Build history of the part. All positions in model axes, mm. A direction names the side the tool comes from. Coordinates: 2 decimals unless noted, no trailing zeros. Order: outer loops, then holes, each group sorted by start corner. A loop starts at its lowest first (then second) coordinate and runs counter-clockwise, first axis right, second up. Notation, with made-up numbers: (20.25, 69.25) - (26.25, 69.25) arc R25 cw to (26.25, 107.25) - close; hole circle Ø7 at (71.5, -5). An arc over 180 degrees is marked (long way). One line per item, written item: value.
from build123d import *

# Parameters (mm, degrees)
SKETCH_1_W              = 26
SKETCH_1_H              = 32.5
HOLE_WIZARD_M39_1_D     = 45
HOLE_WIZARD_M39_1_DEPTH = 10
SKETCH_4_R              = 8
EXTRUDE_1_DEPTH         = 10
CUT_EXTRUDE_1_DEPTH     = 5
SKETCH_6_R              = 1.5
CUT_EXTRUDE_2_DEPTH     = 53.80624963
FILLET_1_R              = 5
FILLET_2_R              = 3


with BuildPart() as part:
    # 草图1 → 旋转1 (revolve)
    with BuildSketch(Plane(origin=(0, 0, 0), x_dir=(-1, 0, 0), z_dir=(0, 0, -1)), mode=Mode.PRIVATE) as revolve_1_sk:
        with Locations((-13, 16.25)):
            Rectangle(SKETCH_1_W, SKETCH_1_H)
    revolve(revolve_1_sk.sketch.rotate(Axis((26, 0, 0), (-1, 0, 0)), 270), axis=Axis((26, 0, 0), (-1, 0, 0)))

    # M39 间隙孔1
    with Locations(Plane(origin=(26, 0, 0), x_dir=(0, 0, -1), z_dir=(1, 0, 0))):
        with Locations((0, 0)):
            Hole(HOLE_WIZARD_M39_1_D / 2, depth=HOLE_WIZARD_M39_1_DEPTH)

    # 草图4 → 凸台-拉伸1 (add)
    with BuildSketch(Plane(origin=(16, 0, 0), x_dir=(0, 0, -1), z_dir=(1, 0, 0))):
        with Locations(Location((0, 0, 0), (0, 0, 180))):
            Circle(SKETCH_4_R)
    extrude(amount=EXTRUDE_1_DEPTH)

    # 草图5 → 切除-拉伸1 (cut)
    with BuildSketch(Plane(origin=(26, 0, 0), x_dir=(0, 0, -1), z_dir=(1, 0, 0))):
        Polygon((3.464101615, -6), (6.92820323, 0), (3.464101615, 6), (-3.464101615, 6), (-6.92820323, 0), (-3.464101615, -6), align=None)
    extrude(amount=-CUT_EXTRUDE_1_DEPTH, mode=Mode.SUBTRACT)

    # 草图6 → 切除-拉伸2 (cut, through all)
    with BuildSketch(Plane(origin=(0, 0, 0), x_dir=(0, 0, -1), z_dir=(1, 0, 0))):
        Circle(SKETCH_6_R)
    extrude(amount=CUT_EXTRUDE_2_DEPTH, mode=Mode.SUBTRACT)

    # 圆角1
    fillet_1_edges = [part.edges().sort_by_distance(p)[0] for p in [
        (0, 0, -32.5),
    ]]
    fillet(fillet_1_edges, radius=FILLET_1_R)

    # 圆角2
    fillet_2_edges = [part.edges().sort_by_distance(p)[0] for p in [
        (26, 0, -32.5),
    ]]
    fillet(fillet_2_edges, radius=FILLET_2_R)


solid = part.part
1. Band-saw the part on C-C, the plane x = 3.25. Give the cut face in (y, z), and give its area (3 significant figures).
Values found:
outline: circle Ø64.37 at (0, 0); hole circle Ø3 at (0, 0)
area: 3,250 mm2
2. Two-plate mould, pull along Y, no slides. Class faces 1 (the face through (13.87, 9.76, 31)), 2 (the face through (23.54, -2.96, 5.22)), 3 (the face through (26, -22, 7)): pulls with the +Y half, pulls with the -Y half, needs draft (parallel to the pull), parting line crosses it, or undercut.
Values found:
face 1: parting line crosses it
face 2: undercut
face 3: needs draft
3. Band-saw the part on A-A, the plane z = 0. Give the cut face in (x, y).
Values found:
outline: (0, -27.5) arc R5 ccw to (5, -32.5) - (23, -32.5) arc R3 ccw to (26, -29.5) - (26, -22.5) - (16, -22.5) - (16, -8) - (26, -8) - (26, -6) - (21, -6) - (21, -1.5) - (0, -1.5) - close; (0, 1.5) - (21, 1.5) - (21, 6) - (26, 6) - (26, 8) - (16, 8) - (16, 22.5) - (26, 22.5) - (26, 29.5) arc R3 ccw to (23, 32.5) - (5, 32.5) arc R5 ccw to (0, 27.5) - close
4. 3-axis set-ups, long thin cutter, end or side, ignore diameter. For faces 4 (the face through (24, 6, 0)), 5 (the face through (0, -6, 0)): which of +Z, -Z, +X, -X, +Y, -Y reach the whole face in a straight line?
Values found:
face 4: +X
face 5: +Z, -Z, -X, +Y, -Y
5. Band-saw the part on B-B, the plane x = 11. Give the cut face in (y, z), and give its area (3 significant figures).
Values found:
outline: circle Ø65 at (0, 0); hole circle Ø3 at (0, 0)
area: 3,310 mm2
6. Flat gauge pins, fed straight in: P1, Ø2, axis at x = 20.5, z = 22, coming from the +Y side; P2, Ø10, axis at x = 21.5, z = 10, coming from the +Y side; P3, Ø13.5, axis at y = -10, z = 2, coming from the +X side; P4, Ø1.5, axis at x = 23.5, z = 1, coming from the -Y side. Where does each tip first touch, or does it go through?
Values found:
P1: stops at y = 24.8
P2: stops at y = 32.11
P3: stops at x = 26
P4: stops at y = -32.5
7. Probe line 1 along Y through (x, z) = (19, 0); line 2 along Y through (x, z) = (8.5, 0); line 3 along Y through (x, z) = (18, 3). List the from-to ranges inside material, lowest first.
Values found:
line 1: y = -32.5 to -22.5, -8 to -1.5, 1.5 to 8, 22.5 to 32.5
line 2: y = -32.5 to -1.5, 1.5 to 32.5
line 3: y = -32.36 to -22.3, -7.42 to 7.42, 22.3 to 32.36
